Could you check a few things on this drawing? It's one solid part, dimensions in mm from its lowest x, y, z. A direction names the side the tool comes from. Give positions to 0.01 mm unless a question says otherwise; leave off trailing zeros. Order: outer loops, then holes, each group sorted by start corner. A loop starts at its lowest first (then second) coordinate and runs counter-clockwise, first axis right, second up. Notation, with made-up numbers: M 58,73 L 102,73 A15 cw 102,85 Z; hole C 11,73 d5. An arc over 180 degrees is marked long. One line per item, written item: value. Start each with the question number.
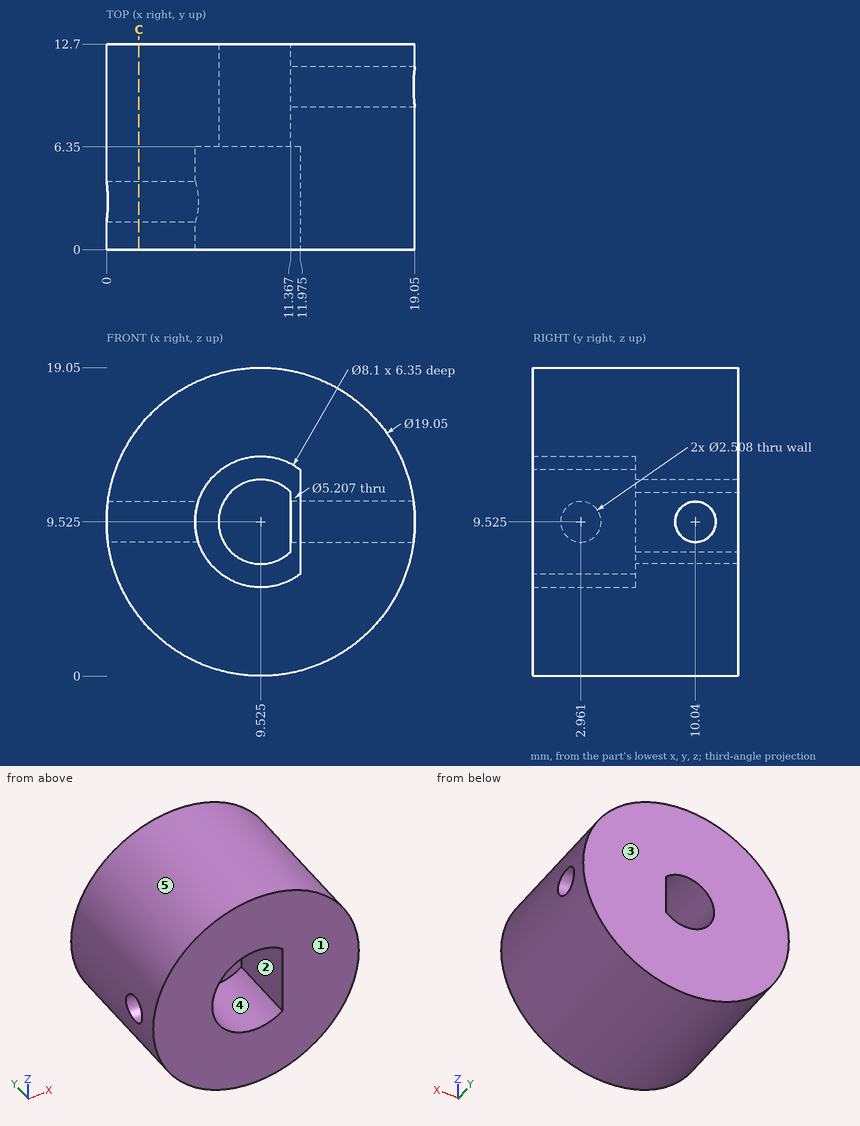
Item 1: I want a section at C-C on x = 2. Write out the boundary of the cut face in (y, z) (1 decimal), plus the area to 3 significant figures.
Item 2: For the marked faces 1 and 2, which set-ups out of +Z, -Z, +X, -X, +Y, -Y let a thin tool reach every point of the face, with its end or its side?
Item 3: Please list where these lines run through material, in increasing order: probe 1 along X at (y, z) = (4.5, 8.25) (1 decimal); probe 2 along Z at (x, y) = (13.25, 10.75); probe 3 along X at (y, z) = (11.5, 7.75) (1 decimal). Write a range as [from, to].
Item 4: Will these pins go through, and if not, where does the flat tip stop? P1, Ø3, axis at y = 4.5, z = 15.5, coming from the -X side; P2, Ø3, axis at x = 10, z = 8.5, coming from the -Y side; P3, Ø1, axis at y = 5, z = 8.5, coming from the +X side (1 decimal); P4, Ø7, axis at x = 9.525, z = 9.525, coming from the -Y side.
Item 5: We'd pull the mould along X, two halves only. Please class the marked faces 3, 4 and 5: +X half, -X half, draft (parallel to the pull), parting line (faces both ways), or undercut.
Answer below:
1. outline: M 0,3.7 L 12.7,3.7 L 12.7,15.4 L 0,15.4 Z; hole C 3,9.5 d2.5
1. area: 143 mm²
2. face 1: +Z, -Z, +X, -X, -Y
2. face 2: -Y
3. probe 1: x = [0.1, 5.7], [12, 19]
3. probe 2: z = [0.76, 8.49], [10.56, 18.29]
3. probe 3: x = [0.2, 7.6], [11.4, 18.9]
4. P1: stops at x = 1.12
4. P2: stops at y = 6.35
4. P3: stops at x = 19
4. P4: stops at y = 0
5. face 3: draft
5. face 4: undercut
5. face 5: parting line
